from build123d import *

# Parameters (mm, degrees)
SKETCH_W     = 137
SKETCH_H     = 73
PAD_DEPTH    = 44
THICKNESS_T  = 3.5
SKETCH001_W  = 36.5
SKETCH001_H  = 23.5
POCKET_DEPTH = 89


with BuildPart() as part:
    # Sketch → Pad (new body)
    with BuildSketch(Plane.XY):
        Rectangle(SKETCH_W, SKETCH_H)
    extrude(amount=PAD_DEPTH)

    # Thickness
    thickness_openings = [part.faces().sort_by_distance(p)[0] for p in [
        (0, 0, 44),
    ]]
    offset(amount=THICKNESS_T, openings=thickness_openings)

    # Sketch001 (on Face12 of Thickness) → Pocket (cut)
    with BuildSketch(Plane.XZ.offset(40)):
        with Locations((53.75, 32.25)):
            Rectangle(SKETCH001_W, SKETCH001_H)
    extrude(amount=-POCKET_DEPTH, mode=Mode.SUBTRACT)


solid = part.part
Could you check a few things on this model? Use its own coordinates, in mm. A direction names the side the tool comes from. Give positions to 0.01 mm unless a question says otherwise; leave off trailing zeros. Order: outer loops, then holes, each group sorted by start corner. A loop starts at its lowest first (then second) coordinate and runs counter-clockwise, first axis right, second up. Notation, with made-up numbers: (2, -26.5) - (28, -26.5) arc R26 cw to (28, 3.5) - close; hole circle Ø5 at (29.5, 9). An arc over 180 degrees is marked (long way). Return JSON: item names as keys, results as strings. Group by question number.
Q1. Will these pins go through, and if not, where does the flat tip stop? pin 1 Ø10 at (y, z) = (23, 39) entering from +X; pin 2 Ø1 at (y, z) = (-37.5, 29.5) entering from +X; pin 3 Ø11 at (x, y) = (60, 10) entering from +Z.
Q2. Thinking about a two-plate mould opening in X: for faces 4 (the face through (-71, 0.51, -2.45)), 5 (the face through (-1, 36.5, 22)), 6 (the face through (-1, 40, 22)), which applies, pulls with the +X half, pulls with the -X half, needs draft (parallel to the pull), parting line crosses it, or undercut?
Q3. Suppose I cut it at C-C, the plane z = 34. Please give me the cut outline in (x, y), and give its area (3 significant figures).
Q4. Suppose I cut it at B-B, the plane y = 24. Please give me the cut outline in (x, z), and give its area (3 significant figures).
Q5. Please list where these lines run through material, in increasing order: line 1 along X through (y, z) = (26, 11); line 2 along Y through (x, z) = (-38, 12.5); line 3 along Z through (x, y) = (-52, 6.5). Write a range as [from, to].
Q6. Suppose I cut it at A-A, the plane z = 4. Please give me the cut outline in (x, y).
Q7. Which directions (+Z, -Z, +X, -X, +Y, -Y) give clear straight access to the entire face, cutting with the end or side of a thin tool? Please do faces 1 (the face through (35.5, -38, 32)), 2 (the face through (71, 0.51, -2.45)), 3 (the face through (-68.5, -1, 22)).
Resolved:
{
 "1": {"pin 1": "stops at x = -68.5", "pin 2": "stops at x = 35.5", "pin 3": "stops at z = 0"},
 "2": {"face 4": "pulls with the -X half", "face 5": "undercut", "face 6": "needs draft"},
 "3": {"outline": "(-72, -36.5) arc R3.5 ccw to (-68.5, -40) - (35.5, -40) - (35.5, -36.5) - (-68.5, -36.5) - (-68.5, 36.5) - (35.5, 36.5) - (35.5, 40) - (-68.5, 40) arc R3.5 ccw to (-72, 36.5) - close", "area": "1,000 mm2"},
 "4": {"outline": "(-72, 0) arc R3.5 ccw to (-68.5, -3.5) - (68.5, -3.5) arc R3.5 ccw to (72, 0) - (72, 20.5) - (68.5, 20.5) - (68.5, 0) - (-68.5, 0) - (-68.5, 44) - (-72, 44) - close", "area": "724 mm2"},
 "5": {"line 1": "x = [-72, -68.5], [68.5, 72]", "line 2": "y = [-40, -36.5], [36.5, 40]", "line 3": "z = [-3.5, 0]"},
 "6": {"outline": "(-72, -36.5) arc R3.5 ccw to (-68.5, -40) - (68.5, -40) arc R3.5 ccw to (72, -36.5) - (72, 36.5) arc R3.5 ccw to (68.5, 40) - (-68.5, 40) arc R3.5 ccw to (-72, 36.5) - close; hole (-68.5, -36.5) - (68.5, -36.5) - (68.5, 36.5) - (-68.5, 36.5) - close"},
 "7": {"face 1": "+Z, +X, +Y, -Y", "face 2": "-Z, +X, +Y, -Y", "face 3": "+Z"}
}
